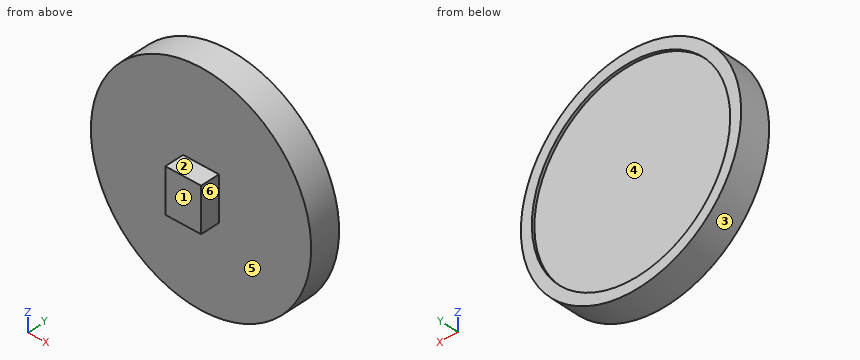
```python
from build123d import *

# Parameters (mm, degrees)
IZIM1_R                     = 40
Y_KSEKLIK_EKSTR_ZYON1_DEPTH = 11
IZIM2_R                     = 36
KES_EKSTR_ZYON2_DEPTH       = 1
IZIM3_W                     = 13
IZIM3_H                     = 16
Y_KSEKLIK_EKSTR_ZYON2_DEPTH = 7


with BuildPart() as part:
    # Çizim1 → Yükseklik-Ekstrüzyon1 (new body)
    with BuildSketch(Plane(origin=(0, 0, 0), x_dir=(1, 0, 0), z_dir=(0, 1, 0))):
        with Locations(Location((-6.982132923, 12.924373709, 0), (0, 0, 270))):
            Circle(IZIM1_R)
    extrude(amount=Y_KSEKLIK_EKSTR_ZYON1_DEPTH)

    # Çizim2 → Kes-Ekstrüzyon2 (cut)
    with BuildSketch(Plane(origin=(0, 11, 0), x_dir=(1, 0, 0), z_dir=(0, 1, 0))):
        with Locations(Location((-6.982132923, 12.924373709, 0), (0, 0, 270))):
            Circle(IZIM2_R)
    extrude(amount=-KES_EKSTR_ZYON2_DEPTH, mode=Mode.SUBTRACT)

    # Çizim3 → Yükseklik-Ekstrüzyon2 (add)
    with BuildSketch(Plane.XZ):
        with Locations((-6.982132923, -12.924373709)):
            Rectangle(IZIM3_W, IZIM3_H)
    extrude(amount=Y_KSEKLIK_EKSTR_ZYON2_DEPTH)


solid = part.part
```
CAD build for the part. Positions are in the model's coordinates, mm. Face numbers are marked on the shaded views. A direction names the side the tool comes from. Coordinates: 2 decimals unless noted, no trailing zeros. Order: outer loops, then holes, each group sorted by start corner. A loop starts at its lowest first (then second) coordinate and runs counter-clockwise, first axis right, second up.
(1) Saw through at D-D, the plane z = -13. Write the cut outline in (x, y).
Solution:
outline: (-46.98, 0) - (-13.48, 0) - (-13.48, -7) - (-0.48, -7) - (-0.48, 0) - (33.02, 0) - (33.02, 11) - (29.02, 11) - (29.02, 10) - (-42.98, 10) - (-42.98, 11) - (-46.98, 11) - close
(2) Saw through at C-C, the plane y = -5.25. Write the cut outline in (x, z).
Solution:
outline: (-13.48, -20.92) - (-0.48, -20.92) - (-0.48, -4.92) - (-13.48, -4.92) - close
(3) Pin check, flat tips, straight feed: pin 1 Ø2 at (x, y) = (-10, -5) entering from +Z; pin 2 Ø3 at (x, z) = (-33, -16) entering from +Y; pin 3 Ø3.5 at (y, z) = (-4, -9.5) entering from -X. Stop position of each tip, or through.
Solution:
pin 1: stops at z = -4.92
pin 2: stops at y = 10
pin 3: stops at x = -13.48
(4) Which spindle directions (+Z, -Z, +X, -X, +Y, -Y) get a long thin tool onto all of the face, cutting with end or side? Do the marked faces 1 and 2. Say none if no direction does.
Solution:
face 1: +Z, -Z, +X, -X, -Y
face 2: +Z, +X, -X, -Y
(5) Saw through at B-B, the plane x = 3. Write the cut outline in (y, z), and give its area (3 significant figures).
Solution:
outline: (0, -51.66) - (11, -51.66) - (11, -47.51) - (10, -47.51) - (10, 21.66) - (11, 21.66) - (11, 25.81) - (0, 25.81) - close
area: 783 mm2
(6) Saw through at A-A, the plane z = -27. Write the cut outline in (x, y), and give its area (3 significant figures).
Solution:
outline: (-44.42, 0) - (30.46, 0) - (30.46, 11) - (26.15, 11) - (26.15, 10) - (-40.12, 10) - (-40.12, 11) - (-44.42, 11) - close
area: 757 mm2
(7) Mould opens along X. For the marked faces 3, 4, 5 and 6 say: released by +X, released by -X, zero draft, split by the parting line, or undercut.
Solution:
face 3: split by the parting line
face 4: undercut
face 5: zero draft
face 6: released by +X
(8) Drill centre lines: L1, parallel to Y at x = -36, z = -14; L2, parallel to Y at x = -23, z = -48.5; L3, parallel to Z at x = 17, y = 5.25. Where is each one in solid material? Low to high.
Solution:
L1: y = 0 to 10
L2: y = 0 to 11
L3: z = -44.94 to 19.09
